from build123d import *

# Parameters (mm, degrees)
SKETCH8_R            = 25
BOSS_EXTRUDE7_DEPTH  = 6
SKETCH11_R           = 5.5
BOSS_EXTRUDE12_DEPTH = 10
SKETCH14_W           = 30
SKETCH14_H           = 10
CUT_EXTRUDE2_DEPTH   = 41.620192023


with BuildPart() as part:
    # Sketch8 → Boss-Extrude7 (new body)
    with BuildSketch(Plane(origin=(0, 0, 0), x_dir=(1, 0, 0), z_dir=(0, 1, 0))):
        with Locations(Location((0, 0, 0), (0, 0, 270))):
            Circle(SKETCH8_R)
    extrude(amount=BOSS_EXTRUDE7_DEPTH)

    # Sketch11 → Boss-Extrude12 (add, symmetric)
    with BuildSketch(Plane.XY):
        with BuildLine():
            Line((20, 6), (-20, 6))
            ThreePointArc((-20, 6), (0, 26), (20, 6))
        make_face()
        with Locations((0, 16)):
            Circle(SKETCH11_R, mode=Mode.SUBTRACT)
    extrude(amount=BOSS_EXTRUDE12_DEPTH, both=True)

    # Sketch14 → Cut-Extrude2 (cut, through all)
    with BuildSketch(Plane(origin=(0, 6, 0), x_dir=(1, 0, 0), z_dir=(0, 1, 0))):
        Rectangle(SKETCH14_W, SKETCH14_H)
    extrude(amount=CUT_EXTRUDE2_DEPTH, mode=Mode.SUBTRACT)

    # Sketch15 → Revolve1 (revolve)
    with BuildSketch(Plane.XY, mode=Mode.PRIVATE) as revolve1_sk:
        with BuildLine():
            Line((0, 0), (0, -25))
            ThreePointArc((0, -25), (17.67766953, -17.67766953), (25, 0))
            Line((25, 0), (0, 0))
        make_face()
    revolve(revolve1_sk.sketch.rotate(Axis((0, 0, 0), (0, -1, 0)), 180), axis=Axis((0, 0, 0), (0, -1, 0)))


solid = part.part
Model file for the job. Use its own axes, mm. A direction names the side the tool comes from. Give positions to 0.01 mm unless a question says otherwise; leave off trailing zeros. Loops run counter-clockwise (first coordinate to the right, second up) from the corner with the lowest first, then second, coordinate; pieces in that order, holes last.
1) Tool access for faces 1 (the cylindrical face through (0, 26, 7)), 2 (the flat face through (0, 9, 10)), 3 (the cylindrical face through (-1.19, 10.63, 7.46)), 4 (the flat face through (-4, 11, -5)), 5 (the flat face through (0, 9, -10)): list every direction of +Z, -Z, +X, -X, +Y, -Y with a clear straight run to the whole face (end or side of a thin tool).
2) Saw through at D-D (y = 9.5). Write the cut outline in (x, z).
3) Saw through at C-C (y = 20). Write the cut outline in (x, z).
4) Flat gauge pins, fed straight in: pin 1 Ø10 at (x, y) = (3.5, -10.5) entering from +Z; pin 2 Ø12.5 at (x, y) = (0, 16) entering from -Z; pin 3 Ø2 at (y, z) = (-12.5, 10) entering from -X. Where does each tip first touch, or does it go through?
5) Saw through at B-B (z = 7). Write the cut outline in (x, y).
6) Pull direction X, two halves, no side cores. Call faces 6 (the flat face through (15, 13, 0)), 7 (the flat face through (0, 6, 11)), 8 (the cylindrical face through (7.509, 2.958, 23.846)): +X half, -X half, draft (parallel to the pull), parting line (faces both ways), or undercut.
7) Wall check: line 1 (Z direction, x = -12, y = 12); line 2 (Y direction, x = 0, z = -7); line 3 (X direction, y = 16, z = -6.35). Give the ranges that are in metal, low to high.
8) Saw through at A-A (x = 0). Write the cut outline in (y, z).
Answer block:
1. face 1: +Z, -Z, +Y
1. face 2: +Z, +X, -X, +Y
1. face 3: +Z, -Z
1. face 4: +Y
1. face 5: -Z, +X, -X, +Y
2. outline: (-19.69, -10) - (19.69, -10) - (19.69, 10) - (-19.69, 10) - close; hole (-15, -5) - (15, -5) - (15, 5) - (-15, 5) - close
3. outline: (-14.28, -10) - (-3.77, -10) - (-3.77, -5) - (-14.28, -5) - close; (-14.28, 5) - (-3.77, 5) - (-3.77, 10) - (-14.28, 10) - close; (3.77, -10) - (14.28, -10) - (14.28, -5) - (3.77, -5) - close; (3.77, 5) - (14.28, 5) - (14.28, 10) - (3.77, 10) - close
4. pin 1: stops at z = 24.25
4. pin 2: stops at z = -10
4. pin 3: stops at x = -19.99
5. outline: (-24, 0) arc R24 ccw to (24, 0) - (24, 6) - (20, 6) arc R20 ccw to (-20, 6) - (-24, 6) - close; hole circle Ø11 at (0, 16)
6. face 6: undercut
6. face 7: draft
6. face 8: parting line
7. line 1: z = -10 to -5, 5 to 10
7. line 2: y = -24 to 10.5, 21.5 to 26
7. line 3: x = -17.32 to -5.5, 5.5 to 17.32
8. outline: (0, -25) - (6, -25) - (6, -10) - (10.5, -10) - (10.5, -5) - (6, -5) - (6, 5) - (10.5, 5) - (10.5, 10) - (6, 10) - (6, 25) - (0, 25) arc R25 ccw to start; (21.5, -10) - (26, -10) - (26, -5) - (21.5, -5) - close; (21.5, 5) - (26, 5) - (26, 10) - (21.5, 10) - close
